For this review, take the finished solid that the model builds, in its own axes (mm). Face numbers are marked on the shaded views. A direction names the side the tool comes from. Give positions to 0.01 mm unless a question says otherwise; leave off trailing zeros. Order: outer loops, then holes, each group sorted by start corner. A loop starts at its lowest first (then second) coordinate and runs counter-clockwise, first axis right, second up. Notation, with made-up numbers: M 69,20 L 101,20 A16 cw 101,33 Z; hole C -39.5,-36.5 d4. An arc over 180 degrees is marked long. Use CSV: the item, a comma, the result in double quotes. Start each with the question number.
(1) Consider section C-C (x = -14.5). Write out the cut boundary in (y, z), and give its area (3 significant figures).
(2) Tool access review of the marked faces 1, 2 and 3: name each direction out of +Z, -Z, +X, -X, +Y, -Y from which nothing blocks a thin tool from reaching the whole face with its end or side.
(3) Consider section B-B (x = -31). Write out the cut boundary in (y, z), and give its area (3 significant figures).
(4) Clearance check with flat-ended pins moving along their axes: P1, Ø5, axis at y = -3.5, z = 3.5, coming from the -X side; P2, Ø3, axis at x = -38.82, y = 0, coming from the -Z side; P3, Ø1.5, axis at x = 11, z = -4, coming from the +Y side; P4, Ø4, axis at x = 31.18, y = 0, coming from the -Z side. State where each tip first meets the part, or that it passes through.
(5) Wall thickness on L1, parallel to X at y = 0, z = 2.5; L2, parallel to X at y = 1, z = 6.5; L3, parallel to X at y = -5, z = -2.5: over which ranges is each line inside the solid? List them lowest first. Write a range as from..to.
(6) Consider section A-A (y = 0). Give the number of separate pieces and of enclosed holes in the cut face, and give its area (3 significant figures).
```python
from build123d import *

# Parameters (mm, degrees)
CHAMFER1_SIZE           = 1
SKETCH2_R               = 1.2
CUT_EXTRUDE1_DEPTH      = 9
CUT_EXTRUDE1_DEPTH_BACK = 9


with BuildPart() as part:
    # Sketch1 → Revolve1 (revolve)
    with BuildSketch(Plane.XY):
        Polygon((-41.319098712, 0), (-41.319098712, 4.5), (-28.333497823, 4.5), (-28.319098712, 5.999930887), (-23.319098712, 5.999930887), (-23.319098712, 8), (15.680901288, 8), (15.680901288, 5), (20.680901288, 5), (20.680901288, 3.95), (38.680901288, 3.95), (38.680901288, 0), align=None)
    revolve(axis=Axis((-41.319098712, 0, 0), (1, 0, 0)))

    # Chamfer1
    chamfer1_edges = [part.edges().sort_by_distance(p)[0] for p in [
        (-41.319098712, -4.5, 0),
        (38.680901288, -3.95, 0),
    ]]
    chamfer(chamfer1_edges, length=CHAMFER1_SIZE)

    # Sketch2 → Cut-Extrude1 (cut, two sides)
    with BuildSketch(Plane.XY) as cut_extrude1_sk:
        with Locations((-38.819098712, 0)):
            Circle(SKETCH2_R)
        with Locations((31.180901288, 0)):
            Circle(SKETCH2_R)
    extrude(amount=CUT_EXTRUDE1_DEPTH, mode=Mode.SUBTRACT)
    extrude(cut_extrude1_sk.sketch, amount=-CUT_EXTRUDE1_DEPTH_BACK, mode=Mode.SUBTRACT)


solid = part.part
```
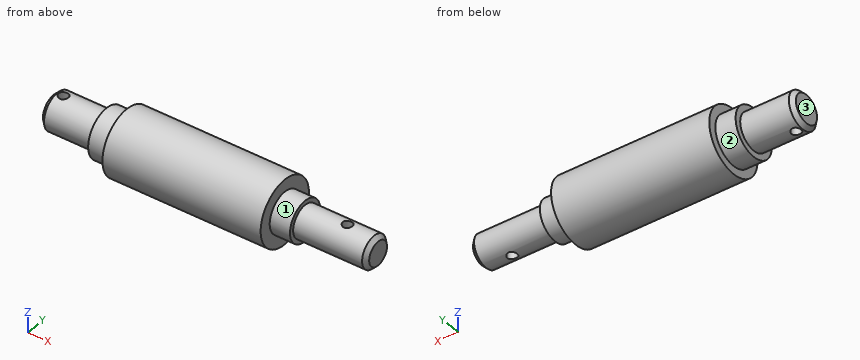
Check result:
1,outline,"C 0,0 d16"
1,area,"201 mm^2"
2,face 1,"+X"
2,face 2,"-X"
2,face 3,"+Z, -Z, -X, +Y, -Y"
3,outline,"C 0,0 d9"
3,area,"63.6 mm^2"
4,P1,"stops at x = -41.32"
4,P2,"stops at z = -4.5"
4,P3,"stops at y = 7.31"
4,P4,"stops at z = -3.95"
5,L1,"x = -41.32..-40.02, -37.62..29.98, 32.38..38.68"
5,L2,"x = -23.32..15.68"
5,L3,"x = -28.32..15.68"
6,separate pieces,"3"
6,enclosed holes,"0"
6,area,"951 mm^2"
